The model under review builds one solid part; all positions refer to its coordinate system, in mm. Round coordinates to 2 decimals unless told otherwise and drop trailing zeros. Order: outer loops, then holes, each group sorted by start corner. A loop starts at its lowest first (then second) coordinate and runs counter-clockwise, first axis right, second up. Notation, with made-up numbers: (-1.75, 57.25) -> (26.25, 57.25) arc R26 cw to (26.25, 82.25) -> close; hole circle Ø10 at (80, -31.75). An arc over 180 degrees is marked (long way). Use a Markdown table: item, result. Add a question column.
```python
from build123d import *

# Parameters (mm, degrees)
SKETCH1_R           = 1.5
BOSS_EXTRUDE1_DEPTH = 1.5
SKETCH3_W           = 2
SKETCH3_H           = 27
BOSS_EXTRUDE2_DEPTH = 4
FILLET1_R           = 1


with BuildPart() as part:
    # Sketch1 → Boss-Extrude1 (new, symmetric)
    with BuildSketch(Plane(origin=(0, 0, 0), x_dir=(1, 0, 0), z_dir=(0, 1, 0))):
        with BuildLine():
            Line((-2.821661699, 1.018933391), (3.310390132, 18))
            ThreePointArc((3.310390132, 18), (3.606995734, 18.973968595), (3.803029904, 19.973048328))
            Line((3.803029904, 19.973048328), (7.689609868, 47))
            Line((7.689609868, 47), (8.050720979, 48))
            Line((8.050720979, 48), (11.689609868, 48))
            Line((11.689609868, 48), (11.689609868, 18))
            Line((11.689609868, 18), (9.689609868, 18))
            Line((9.689609868, 18), (2.821661699, -1.018933391))
            ThreePointArc((2.821661699, -1.018933391), (-1.018933391, -2.821661699), (-2.821661699, 1.018933391))
        make_face()
        with Locations(Location((6.5, 18, 0), (0, 0, 270))):
            Circle(SKETCH1_R, mode=Mode.SUBTRACT)
        with Locations(Location((0, 0, 0), (0, 0, 270))):
            Circle(SKETCH1_R, mode=Mode.SUBTRACT)
    extrude(amount=BOSS_EXTRUDE1_DEPTH, both=True)

    # Sketch3 → Boss-Extrude2 (add, symmetric)
    with BuildSketch(Plane(origin=(0, 0, 0), x_dir=(1, 0, 0), z_dir=(0, 1, 0))):
        with Locations((11.689609868, 34.5)):
            Rectangle(SKETCH3_W, SKETCH3_H)
    extrude(amount=BOSS_EXTRUDE2_DEPTH, both=True)

    # Fillet1
    fillet1_edges = [part.edges().sort_by_distance(p)[0] for p in [
        (11.689609868, -4, -48),
        (11.689609868, -4, -21),
        (11.689609868, 4, -48),
        (11.689609868, 4, -21),
    ]]
    fillet(fillet1_edges, radius=FILLET1_R)


solid = part.part
```
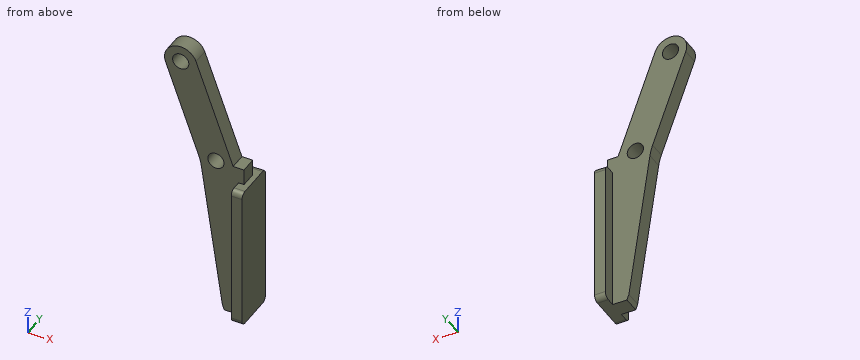
Q1. Add section D-D (z = -23). Write out the cut boundary in (x, y).
Q2. Add section C-C (x = -0.5). Write out the cut boundary in (y, z), then the cut area to 3 significant figures.
Q3. Add section B-B (z = 0). Write out the cut boundary in (x, y).
Q4. Insertion check: pin 1 (1.6 mm diameter, centred on x = 12, y = 0, fed in from +Z); pin 2 (5 mm diameter, centred on x = 0, z = 0, fed in from -Y); pin 3 (3.5 mm diameter, centred on y = -0.5, z = -19, fed in from +X). Each pin has a flat end and moves straight along its axis. Give the tip position at first contact, or say it passes through.
Q5. Add section A-A (y = 0). Write out the cut boundary in (x, z), then the cut area to 3 significant figures.
Q6. Wall thickness on line 1 (Y direction, x = 8.25, z = -25); line 2 (X direction, y = -3.5, z = -36); line 3 (X direction, y = 1, z = -0.5): over which ranges is each line inside the solid? List them lowest first. Write a range as [from, to].
Report:
| question | item | result |
|---|---|---|
| 1 | outline | (4.24, -1.5) -> (10.69, -1.5) -> (10.69, -4) -> (12.69, -4) -> (12.69, 4) -> (10.69, 4) -> (10.69, 1.5) -> (4.24, 1.5) -> close |
| 2 | outline | (-1.5, -7.45) -> (1.5, -7.45) -> (1.5, -1.41) -> (-1.5, -1.41) -> close; (-1.5, 1.41) -> (1.5, 1.41) -> (1.5, 2.96) -> (-1.5, 2.96) -> close |
| 2 | area | 22.7 mm² |
| 3 | outline | (-3, -1.5) -> (-1.5, -1.5) -> (-1.5, 1.5) -> (-3, 1.5) -> close; (1.5, -1.5) -> (3.19, -1.5) -> (3.19, 1.5) -> (1.5, 1.5) -> close |
| 4 | pin 1 | stops at z = -18 |
| 4 | pin 2 | stops at y = -1.5 |
| 4 | pin 3 | stops at x = 11.69 |
| 5 | outline | (-2.82, -1.02) -> (3.31, -18) arc R10 cw to (3.8, -19.97) -> (7.69, -47) -> (8.05, -48) -> (12.69, -48) -> (12.69, -21) -> (11.69, -21) -> (11.69, -18) -> (9.69, -18) -> (2.82, 1.02) arc R3 ccw to start; hole circle Ø3 at (0, 0); hole circle Ø3 at (6.5, -18) |
| 5 | area | 322 mm² |
| 6 | line 1 | y = [-1.5, 1.5] |
| 6 | line 2 | x = [10.69, 12.69] |
| 6 | line 3 | x = [-2.96, -1.41], [1.41, 3.37] |
